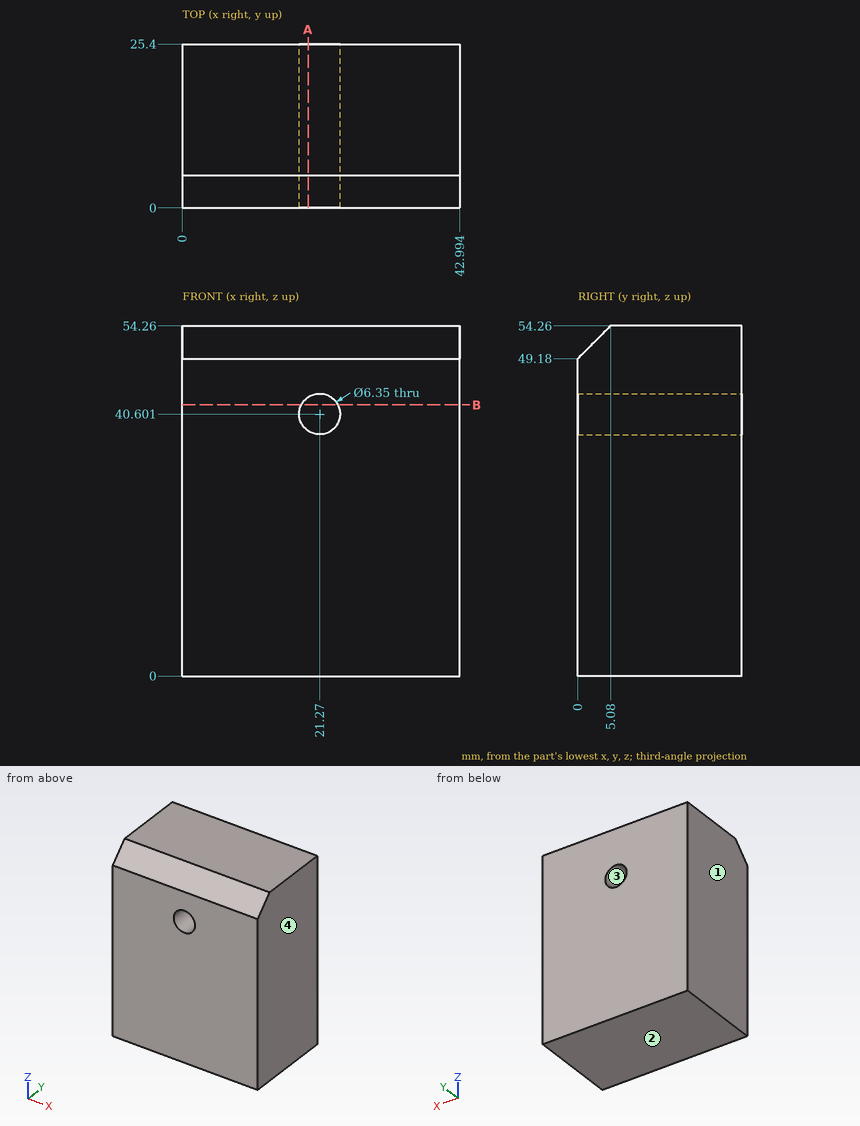
Geometry: see drawing. Coordinates: mm, zero at the bounding-box minimum. Coordinates: 2 decimals unless noted, no trailing zeros. Loops run counter-clockwise (first coordinate to the right, second up) from the corner with the lowest first, then second, coordinate; pieces in that order, holes last. Notation, with made-up numbers: (15, 77) - (22, 77) arc R24 cw to (22, 89) - close; hole circle Ø8 at (76.25, 15.25). An arc over 180 degrees is marked (long way). Put each result on its own line as item: value. Start each with the question number.
Q1. Line query: line 1 (X direction, y = 24, z = 40.5); line 2 (Y direction, x = 17, z = 50); line 3 (Y direction, x = 21, z = 50.5). Output: solid intervals per line, ascending.
Q2. Pull-direction query (X, two-part tool) for the marked faces 1, 2, 3 and 4; classes: released by +X, released by -X, zero draft, split by the parting line, or undercut.
Q3. Cut plane B-B, the plane z = 42. Return loops of the section in (x, y).
Q4. Cut plane A-A, the plane x = 19.5. Return loops of the section in (y, z) (1 decimal).
Q5. Pin query (flat end, axial travel): pin 1 Ø8 at (y, z) = (22.5, 47.5) entering from -X; pin 2 Ø5 at (x, z) = (21.27, 40.6) entering from +Y. Return the tip coordinate at first contact, or that it passes through.
Filled sheet:
1. line 1: 0 to 18.1, 24.44 to 42.99
1. line 2: 0.82 to 25.4
1. line 3: 1.32 to 25.4
2. face 1: released by -X
2. face 2: zero draft
2. face 3: undercut
2. face 4: released by +X
3. outline: (0, 0) - (18.42, 0) - (18.42, 25.4) - (0, 25.4) - close; (24.12, 0) - (42.99, 0) - (42.99, 25.4) - (24.12, 25.4) - close
4. outline: (0, 0) - (25.4, 0) - (25.4, 38) - (0, 38) - close; (0, 43.2) - (25.4, 43.2) - (25.4, 54.3) - (5.1, 54.3) - (0, 49.2) - close
5. pin 1: x = 0
5. pin 2: through
